from build123d import *

# Parameters (mm, degrees)
SKETCH1_W                      = 60.3
SKETCH1_H                      = 35
BOSS_EXTRUDE1_DEPTH            = 40
SKETCH2_W                      = 47
SKETCH2_H                      = 25
SKETCH2_W_2                    = 54.3
SKETCH2_H_2                    = 8
SKETCH2_W_3                    = 4.65
SKETCH2_H_3                    = 23
CUT_EXTRUDE1_DEPTH             = 54.059141531
M3_CLEARANCE_HOLE2_D           = 3.4
M3_CLEARANCE_HOLE2_DEPTH       = 2
M3_CLEARANCE_HOLE2_CSINK_D     = 3.45
M3_CLEARANCE_HOLE2_CSINK_ANGLE = 90
M3_CLEARANCE_HOLE3_D           = 3.4
M3_CLEARANCE_HOLE3_DEPTH       = 2
M3_CLEARANCE_HOLE3_CSINK_D     = 3.45
M3_CLEARANCE_HOLE3_CSINK_ANGLE = 90


with BuildPart() as part:
    # Sketch1 → Boss-Extrude1 (new body)
    with BuildSketch(Plane.XY):
        Rectangle(SKETCH1_W, SKETCH1_H)
    extrude(amount=BOSS_EXTRUDE1_DEPTH)

    # Sketch2 → Cut-Extrude1 (cut, through all)
    with BuildSketch(Plane(origin=(0, 0, 0), x_dir=(-1, 0, 0), z_dir=(0, 0, -1))):
        with Locations((0, -5)):
            Rectangle(SKETCH2_W, SKETCH2_H)
        with Locations((0, 13.5)):
            Rectangle(SKETCH2_W_2, SKETCH2_H_2)
        with Locations((-27.825, -4)):
            Rectangle(SKETCH2_W_3, SKETCH2_H_3)
        with Locations((27.825, -4)):
            Rectangle(SKETCH2_W_3, SKETCH2_H_3)
    extrude(amount=-CUT_EXTRUDE1_DEPTH, mode=Mode.SUBTRACT)

    # M3 Clearance Hole2
    with Locations(Plane(origin=(0, -15.5, 0), x_dir=(1, 0, 0), z_dir=(0, 1, 0))):
        with Locations((-27.82, -20)):
            CounterSinkHole(M3_CLEARANCE_HOLE2_D / 2, M3_CLEARANCE_HOLE2_CSINK_D / 2, depth=M3_CLEARANCE_HOLE2_DEPTH, counter_sink_angle=M3_CLEARANCE_HOLE2_CSINK_ANGLE)

    # M3 Clearance Hole3
    with Locations(Plane(origin=(0, -15.5, 0), x_dir=(1, 0, 0), z_dir=(0, 1, 0))):
        with Locations((27.82, -20)):
            CounterSinkHole(M3_CLEARANCE_HOLE3_D / 2, M3_CLEARANCE_HOLE3_CSINK_D / 2, depth=M3_CLEARANCE_HOLE3_DEPTH, counter_sink_angle=M3_CLEARANCE_HOLE3_CSINK_ANGLE)


solid = part.part
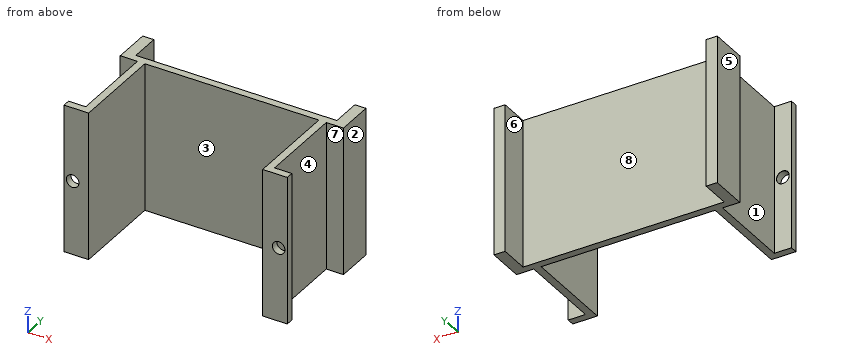
Design review of the part built by this model. Coordinates are the model's own, in mm. Face numbers are marked on the shaded views. A direction names the side the tool comes from. Coordinates: 2 decimals unless noted, no trailing zeros. Order: outer loops, then holes, each group sorted by start corner. A loop starts at its lowest first (then second) coordinate and runs counter-clockwise, first axis right, second up. Notation, with made-up numbers: (28.5, -36.75) -> (54.5, -36.75) arc R24 cw to (54.5, -24.75) -> close; hole circle Ø2 at (-1.5, 44). An arc over 180 degrees is marked (long way). One line per item, written item: value.
1) To check wall thickness, follow probe 1 along X at (y, z) = (-16, 20); probe 2 along Z at (x, y) = (-27.82, -16.95); probe 3 along X at (y, z) = (-3, 26). State the ranges of each line that lie inside material, in increasing order. Write a range as [from, to].
Output values:
probe 1: x = [-30.15, -29.52], [-26.12, -23.5], [23.5, 26.12], [29.52, 30.15]
probe 2: z = [0, 18.3], [21.7, 40]
probe 3: x = [-25.5, -23.5], [23.5, 25.5]
2) Machinability: for the marked faces 1, 2, 3, 4 and 5, which of the approach directions +Z, -Z, +X, -X, +Y, -Y give a long, thin tool a straight path to every point of the face, cutting with its end or side? Answer none if there is none.
Output values:
face 1: +Z, -Z, -X
face 2: +Z, -Z, +X, +Y, -Y
face 3: +Z, -Z, -Y
face 4: +Z, -Z, +X
face 5: +Z, -Z, -X, +Y, -Y
3) We need section D-D, the plane z = 34.5. Give the boundary of the cut face in (x, y), then the cut area to 3 significant figures.
Output values:
outline: (-30.15, -17.5) -> (-23.5, -17.5) -> (-23.5, 7.5) -> (23.5, 7.5) -> (23.5, -17.5) -> (30.15, -17.5) -> (30.15, -15.5) -> (25.5, -15.5) -> (25.5, 7.5) -> (30.15, 7.5) -> (30.15, 17.5) -> (27.15, 17.5) -> (27.15, 9.5) -> (-27.15, 9.5) -> (-27.15, 17.5) -> (-30.15, 17.5) -> (-30.15, 7.5) -> (-25.5, 7.5) -> (-25.5, -15.5) -> (-30.15, -15.5) -> close
area: 287 mm2
4) We need section B-B, the plane x = 27.82. Give the boundary of the cut face in (y, z) (3 decimals).
Output values:
outline: (-17.5, 0) -> (-15.5, 0) -> (-15.5, 18.275) -> (-15.525, 18.3) -> (-17.5, 18.3) -> close; (-17.5, 21.7) -> (-15.525, 21.7) -> (-15.5, 21.725) -> (-15.5, 40) -> (-17.5, 40) -> close; (7.5, 0) -> (17.5, 0) -> (17.5, 40) -> (7.5, 40) -> close
5) We need section A-A, the plane z = 20. Count the separate pieces of the cut face and the enclosed holes in it, then the cut area to 3 significant figures.
Output values:
separate pieces: 3
enclosed holes: 0
area: 274 mm2
6) Draft analysis for pull direction Y (two halves, no side actions). For the marked faces 6, 7 and 8, state which applies: +Y half, -Y half, draft (parallel to the pull), parting line (faces both ways), or undercut.
Output values:
face 6: draft
face 7: undercut
face 8: +Y half
7) Clearance check with flat-ended pins moving along their axes: P1, Ø6, axis at x = 13, z = 14.5, coming from the -Y side; P2, Ø11.5, axis at y = 1.5, z = 24.5, coming from the +X side; P3, Ø3, axis at x = 9.5, z = 17, coming from the +Y side. State where each tip first meets the part, or that it passes through.
Output values:
P1: stops at y = 7.5
P2: stops at x = 25.5
P3: stops at y = 9.5
8) We need section C-C, the plane y = -14. Give the boundary of the cut face in (x, z).
Output values:
outline: (-25.5, 0) -> (-23.5, 0) -> (-23.5, 40) -> (-25.5, 40) -> close; (23.5, 0) -> (25.5, 0) -> (25.5, 40) -> (23.5, 40) -> close
